```python
from build123d import *

# Parameters (mm, degrees)
P_IDAT_VYSUNUT_M1_DEPTH  = 30
SKICA2_R                 = 1.8
ODEBRAT_VYSUNUT_M1_DEPTH = 8
ZAOBLIT1_R               = 1
ZKOSEN_2_SIZE            = 0.25
ZKOSEN_3_SIZE            = 0.5
ZKOSEN_4_SIZE            = 0.5


with BuildPart() as part:
    # Skica1 → Přidat vysunutím1 (new body)
    with BuildSketch(Plane.XY):
        Polygon((0, 0), (9.7, 0), (11.453718229, 2.09), (11.453718229, 2.7), (9.7, 4.79), (9.7, 5.74), (9.95, 5.99), (25.05, 5.99), (25.3, 5.74), (25.3, 4.79), (23.546281771, 2.7), (23.546281771, 2.09), (25.3, 0), (35, 0), (35, 8), (0, 8), align=None)
    extrude(amount=P_IDAT_VYSUNUT_M1_DEPTH)

    # Skica2 → Odebrat vysunutím1 (cut)
    with BuildSketch(Plane(origin=(0, 8, 0), x_dir=(1, 0, 0), z_dir=(0, 1, 0))):
        with Locations(Location((5.5, -5.5, 0), (0, 0, 180))):
            Circle(SKICA2_R)
        with Locations(Location((29.5, -5.5, 0), (0, 0, 180))):
            Circle(SKICA2_R)
        with Locations(Location((5.5, -24.5, 0), (0, 0, 180))):
            Circle(SKICA2_R)
        with Locations(Location((29.5, -24.5, 0), (0, 0, 180))):
            Circle(SKICA2_R)
    extrude(amount=-ODEBRAT_VYSUNUT_M1_DEPTH, mode=Mode.SUBTRACT)

    # Zaoblit1
    zaoblit1_edges = [part.edges().sort_by_distance(p)[0] for p in [
        (35, 4, 0),
        (0, 4, 0),
        (0, 4, 30),
        (35, 4, 30),
    ]]
    fillet(zaoblit1_edges, radius=ZAOBLIT1_R)

    # Zkosení2
    zkosen_2_edges = [part.edges().sort_by_distance(p)[0] for p in [
        (10.576859115, 1.045, 30),
        (11.453718229, 2.395, 30),
        (24.423140885, 1.045, 0),
        (23.546281771, 2.395, 0),
        (24.423140885, 3.745, 0),
        (25.3, 5.265, 0),
        (25.175, 5.865, 0),
        (17.5, 5.99, 0),
        (9.825, 5.865, 0),
        (9.7, 5.265, 0),
        (10.576859115, 3.745, 0),
        (11.453718229, 2.395, 0),
        (10.576859115, 3.745, 30),
        (10.576859115, 1.045, 0),
        (9.7, 5.265, 30),
        (9.825, 5.865, 30),
        (17.5, 5.99, 30),
        (25.175, 5.865, 30),
        (25.3, 5.265, 30),
        (24.423140885, 3.745, 30),
        (23.546281771, 2.395, 30),
        (24.423140885, 1.045, 30),
    ]]
    chamfer(zkosen_2_edges, length=ZKOSEN_2_SIZE)

    # Zkosení3
    zkosen_3_edges = [part.edges().sort_by_distance(p)[0] for p in [
        (17.5, 8, 30),
        (0, 8, 15),
        (17.5, 8, 0),
        (35, 8, 15),
        (34.707106781, 8, 0.292893219),
        (34.707106781, 8, 29.707106781),
        (0.292893219, 8, 0.292893219),
        (0.292893219, 8, 29.707106781),
    ]]
    chamfer(zkosen_3_edges, length=ZKOSEN_3_SIZE)

    # Zkosení4
    zkosen_4_edges = [part.edges().sort_by_distance(p)[0] for p in [
        (31.3, 8, 5.5),
        (7.3, 8, 24.5),
        (31.3, 8, 24.5),
        (7.3, 8, 5.5),
    ]]
    chamfer(zkosen_4_edges, length=ZKOSEN_4_SIZE)


solid = part.part
```
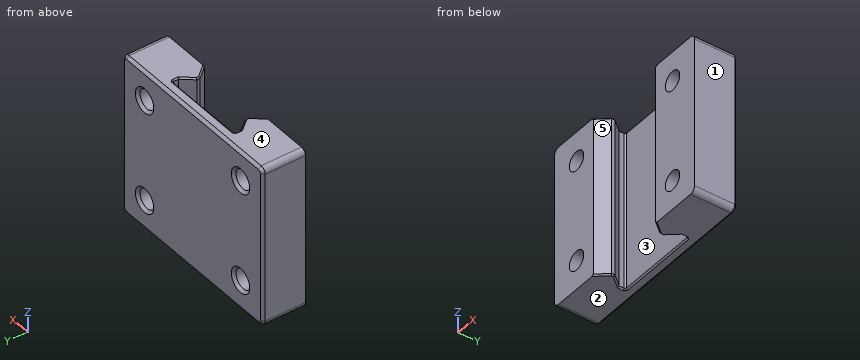
Source: CAD feature listing. Evaluate the final solid. Frame: model axes, mm. Face numbers are marked on the shaded views. A direction names the side the tool comes from. Coordinates: 2 decimals unless noted, no trailing zeros. Order: outer loops, then holes, each group sorted by start corner. A loop starts at its lowest first (then second) coordinate and runs counter-clockwise, first axis right, second up. Notation, with made-up numbers: (63, 50.25) - (97, 50.25) arc R27 cw to (97, 76.25) - close; hole circle Ø3 at (64.5, 68). An arc over 180 degrees is marked (long way). One line per item, written item: value.
1) Ray query, line 1 (Z direction, x = 5.5, y = 5.5); line 2 (X direction, y = 7.25, z = 23); line 3 (Z direction, x = 28, y = 1.75). Return the intervals inside material, ascending. Write a range as [from, to].
Computed values:
line 1: z = [0, 3.7], [7.3, 22.7], [26.3, 30]
line 2: x = [0, 4.51], [6.49, 28.51], [30.49, 35]
line 3: z = [0, 4.51], [6.49, 23.51], [25.49, 30]
2) Cut plane D-D on y = 1. Output: boundary loops of the cut face in (x, z).
Computed values:
outline: (0, 1) arc R1 ccw to (1, 0) - (10.21, 0) - (10.54, 0.25) - (10.54, 29.75) - (10.21, 30) - (1, 30) arc R1 ccw to (0, 29) - close; (24.46, 0.25) - (24.79, 0) - (34, 0) arc R1 ccw to (35, 1) - (35, 29) arc R1 ccw to (34, 30) - (24.79, 30) - (24.46, 29.75) - close; hole circle Ø3.6 at (5.5, 5.5); hole circle Ø3.6 at (5.5, 24.5); hole circle Ø3.6 at (29.5, 5.5); hole circle Ø3.6 at (29.5, 24.5)
3) Cut plane B-B on z = 5.5. State how many separate pieces and enclosed holes the cut face has, plus the area to 3 significant figures.
Computed values:
separate pieces: 3
enclosed holes: 0
area: 138 mm^2
4) Cut plane A-A on x = 29.5. Output: boundary loops of the cut face in (y, z).
Computed values:
outline: (0, 0) - (7.5, 0) - (8, 0.5) - (8, 3.2) - (7.5, 3.7) - (0, 3.7) - close; (0, 7.3) - (7.5, 7.3) - (8, 7.8) - (8, 22.2) - (7.5, 22.7) - (0, 22.7) - close; (0, 26.3) - (7.5, 26.3) - (8, 26.8) - (8, 29.5) - (7.5, 30) - (0, 30) - close
5) Contact query for flat-ended pins moving along their axis: pin 1 (4.5 mm diameter, centred on x = 29.5, z = 5.5, fed in from -Y); pin 2 (4.5 mm diameter, centred on x = 17, z = 17.5, fed in from -Y); pin 3 (1.5 mm diameter, centred on x = 11, z = 24.5, fed in from -Y). Output: stop coordinate, or through.
Computed values:
pin 1: stops at y = 0
pin 2: stops at y = 5.99
pin 3: stops at y = 0.66
6) Reachability of the marked faces 4 and 5 from +Z, -Z, +X, -X, +Y, -Y: full face, straight path, thin tool, end or side. Return the list, or none.
Computed values:
face 4: +Z, +X, -X, +Y, -Y
face 5: +Z, -Z, -Y
7) Mould query, pull axis X, two halves, no side actions, for the marked faces 1, 2 and 3. Classes: released by +X, released by -X, zero draft, split by the parting line, or undercut.
Computed values:
face 1: released by +X
face 2: zero draft
face 3: undercut
8) Cut plane C-C on y = 6.75. Output: boundary loops of the cut face in (x, z).
Computed values:
outline: (0, 1) arc R1 ccw to (1, 0) - (34, 0) arc R1 ccw to (35, 1) - (35, 29) arc R1 ccw to (34, 30) - (1, 30) arc R1 ccw to (0, 29) - close; hole circle Ø3.6 at (5.5, 5.5); hole circle Ø3.6 at (5.5, 24.5); hole circle Ø3.6 at (29.5, 5.5); hole circle Ø3.6 at (29.5, 24.5)
